Autodesk Inventor part; units mm, degrees
ref_plane "YZ Plane" through (0, 0, 0) normal (1, 0, 0) x (0, 1, 0)
ref_plane "XZ Plane" through (0, 0, 0) normal (0, 1, 0) x (-1, 0, 0)
ref_plane "XY Plane" through (0, 0, 0) normal (0, 0, 1) x (1, 0, 0)
sketch "Sketch1" plane through (0, 0, 0) normal (0, 1, 0) x (-1, 0, 0)
  circle A0 centre (0, 0) radius 3.6
  dimension "d0" = 7.2
extrude "Extrusion1" add sketch "Sketch1" along normal blind 2
sketch "Sketch2" plane through (0, 2, 0) normal (0, 1, 0) x (1, 0, 0)
  line L0 (1.7034, 0) -> (0.8517, -1.4752)
  line L1 (0.8517, -1.4752) -> (-0.8517, -1.4752)
  line L2 (-0.8517, -1.4752) -> (-1.7034, 0)
  line L3 (-1.7034, 0) -> (-0.8517, 1.4752)
  line L4 (-0.8517, 1.4752) -> (0.8517, 1.4752)
  line L5 (0.8517, 1.4752) -> (1.7034, 0)
  point P0 (0, 0)
  point P1 (0, 0)
extrude "Extrusion2" cut sketch "Sketch2" against normal blind 1
fillet "Fillet1" radius 1.7 1 edges at (3.6, 2, 0)
sketch "Sketch3" plane through (0, 0, 0) normal (0, -1, 0) x (1, 0, 0)
  circle A0 centre (0, 0) radius 2
  dimension "d6" = 4
extrude "Extrusion3" add sketch "Sketch3" along normal blind 16
thread "Thread1"
chamfer "Chamfer1" distance 0.2 angle 45 1 edges at (-2, -16, 0)
properties part number "Bolt 4 mm x 16 mm"
Design review of the part built by this model. Coordinates are the model's own, in mm. A direction names the side the tool comes from. Give positions to 0.01 mm unless a question says otherwise; leave off trailing zeros. Write each loop counter-clockwise with the first axis right and the second up, starting at its lowest first coordinate (ties: lowest second). Pieces come first, ordered by that corner, then holes.
(1) Tool access review of faces 1 (the face through (0, 1.5, -1.475)), 2 (the face through (0, -16, 0)): name each direction out of +Z, -Z, +X, -X, +Y, -Y from which nothing blocks a thin tool from reaching the whole face with its end or side.
Checked values:
face 1: +Y
face 2: +Z, -Z, +X, -X, -Y
(2) Wall thickness on line 1 along Y through (x, z) = (1.25, 0.25); line 2 along X through (y, z) = (0.75, 2.75); line 3 along Z through (x, y) = (0, -13): over which ranges is each line inside the solid? List them lowest first.
Checked values:
line 1: y = -16 to 1
line 2: x = -2.23 to 2.23
line 3: z = -2 to 2
(3) Mouldability with a two-part tool opening along X and no side actions: class faces 3 (the face through (-2, 0, -2)), 4 (the face through (0, 1.5, 1.475)), 5 (the face through (0, -8, 2)) as +X half, -X half, draft (parallel to the pull), parting line (faces both ways), or undercut.
Checked values:
face 3: draft
face 4: undercut
face 5: parting line
(4) Add section A-A (x = 0). Give the boundary of the cut face in (y, z).
Checked values:
outline: (-16, -1.8) - (-15.8, -2) - (0, -2) - (0, -3.6) - (0.3, -3.6) arc R1.7 ccw to (2, -1.9) - (2, -1.48) - (1, -1.48) - (1, 1.48) - (2, 1.48) - (2, 1.9) arc R1.7 ccw to (0.3, 3.6) - (0, 3.6) - (0, 2) - (-15.8, 2) - (-16, 1.8) - close
(5) Clearance check with flat-ended pins moving along their axes: pin 1 Ø2 at (y, z) = (-14, 2) entering from +X; pin 2 Ø3 at (x, y) = (-1, -4.5) entering from +Z; pin 3 Ø1.5 at (x, z) = (-2.5, 0) entering from -Y; pin 4 Ø0.8 at (x, y) = (0, 1.5) entering from -Z. State where each tip first meets the part, or that it passes through.
Checked values:
pin 1: stops at x = 1.73
pin 2: stops at z = 2
pin 3: stops at y = -16
pin 4: stops at z = -3.4
(6) Add section B-B (y = -10). Give the boundary of the cut face in (x, z).
Checked values:
outline: circle Ø4 at (0, 0)
(7) Add section C-C (y = 0.5). Give the boundary of the cut face in (x, z), and give its area (3 significant figures).
Checked values:
outline: circle Ø7.18 at (0, 0)
area: 40.4 mm2
